Part print with two shaded views. Sizes in mm from the minimum x, y, z corner. Round coordinates to 2 decimals unless told otherwise and drop trailing zeros. Write each loop counter-clockwise with the first axis right and the second up, starting at its lowest first coordinate (ties: lowest second). Pieces come first, ordered by that corner, then holes. Notation, with made-up numbers: M -8,59 L 25,59 A21 ccw 25,72 Z; hole C 84,85.5 d5. An arc over 180 degrees is marked long. One line per question, with ' | ' between items. Start each with the question number.
1) Wall check: probe 1 along Y at (x, z) = (15, 11.5); probe 2 along Y at (x, z) = (15, 1.2); probe 3 along X at (y, z) = (10.75, 10.75). Give the ranges that are in metal, low to high. Write a range as [from, to].
2) Saw through at D-D (z = 12.5). List the corners of the cut face in (x, y).
3) Saw through at A-A (x = 15). List the corners of the cut face in (y, z).
4) Drop flat-ended pins along their axis: pin 1 Ø6 at (x, z) = (26.5, 4.5) entering from -Y; pin 2 Ø5 at (x, z) = (25, 9) entering from -Y; pin 3 Ø1.5 at (x, z) = (18.5, 12.5) entering from +Y. Give the stop position or say it passes through.
5) Mould opens along X. For the marked faces 1, 2 and 3 say: pulls with the +X half, pulls with the -X half, needs draft (parallel to the pull), parting line crosses it, or undercut.
6) Saw through at C-C (y = 11.5). List the corners of the cut face in (x, z), plus the area to 3 significant figures.
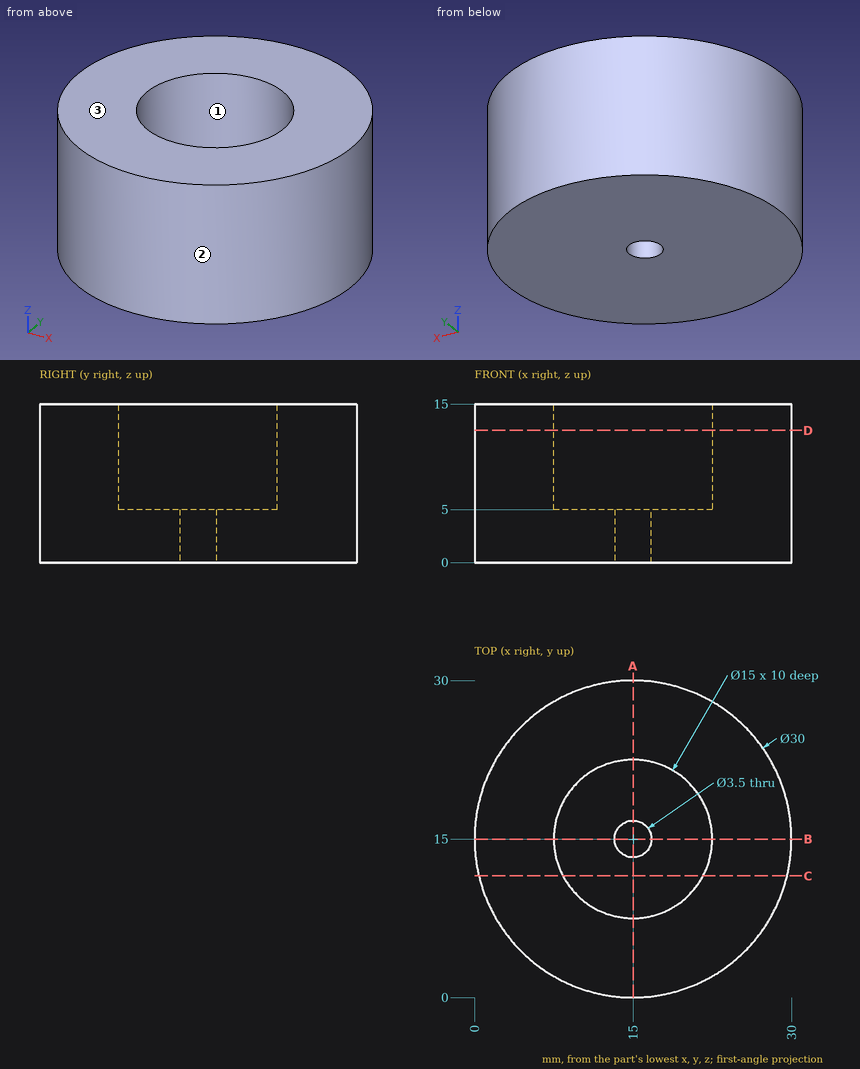
Answer key:
1) probe 1: y = [0, 7.5], [22.5, 30] | probe 2: y = [0, 13.25], [16.75, 30] | probe 3: x = [0.61, 8.82], [21.18, 29.39]
2) outline: C 15,15 d30; hole C 15,15 d15
3) outline: M 0,0 L 13.25,0 L 13.25,5 L 7.5,5 L 7.5,15 L 0,15 Z; M 16.75,0 L 30,0 L 30,15 L 22.5,15 L 22.5,5 L 16.75,5 Z
4) pin 1: stops at y = 2.64 | pin 2: stops at y = 2.01 | pin 3: stops at y = 29.75
5) face 1: undercut | face 2: parting line crosses it | face 3: needs draft
6) outline: M 0.41,0 L 29.59,0 L 29.59,15 L 21.63,15 L 21.63,5 L 8.37,5 L 8.37,15 L 0.41,15 Z | area: 305 mm2
